from build123d import *

# Parameters (mm, degrees)
SKETCH1_W           = 169
SKETCH1_H           = 4
BOSS_EXTRUDE1_DEPTH = 109
SKETCH3_W           = 165
SKETCH3_H           = 105
CUT_EXTRUDE1_DEPTH  = 1.5
SKETCH4_W           = 151
SKETCH4_H           = 91
CUT_EXTRUDE2_DEPTH  = 5
SKETCH5_W           = 84.5
SKETCH5_H           = 1.5
CUT_EXTRUDE3_DEPTH  = 2


with BuildPart() as part:
    # Sketch1 → Boss-Extrude1 (new body)
    with BuildSketch(Plane.XY):
        with Locations((84.5, 2)):
            Rectangle(SKETCH1_W, SKETCH1_H)
    extrude(amount=-BOSS_EXTRUDE1_DEPTH)

    # Sketch3 → Cut-Extrude1 (cut)
    with BuildSketch(Plane.XZ):
        with Locations((84.5, -54.5)):
            Rectangle(SKETCH3_W, SKETCH3_H)
    extrude(amount=-CUT_EXTRUDE1_DEPTH, mode=Mode.SUBTRACT)

    # Sketch4 → Cut-Extrude2 (cut)
    with BuildSketch(Plane(origin=(0, 4, 0), x_dir=(1, 0, 0), z_dir=(0, 1, 0))):
        with Locations((84.5, 54.5)):
            Rectangle(SKETCH4_W, SKETCH4_H)
    extrude(amount=-CUT_EXTRUDE2_DEPTH, mode=Mode.SUBTRACT)

    # Sketch5 → Cut-Extrude3 (cut)
    with BuildSketch(Plane.XY):
        with Locations((84.5, 0.75)):
            Rectangle(SKETCH5_W, SKETCH5_H)
    extrude(amount=-CUT_EXTRUDE3_DEPTH, mode=Mode.SUBTRACT)


solid = part.part
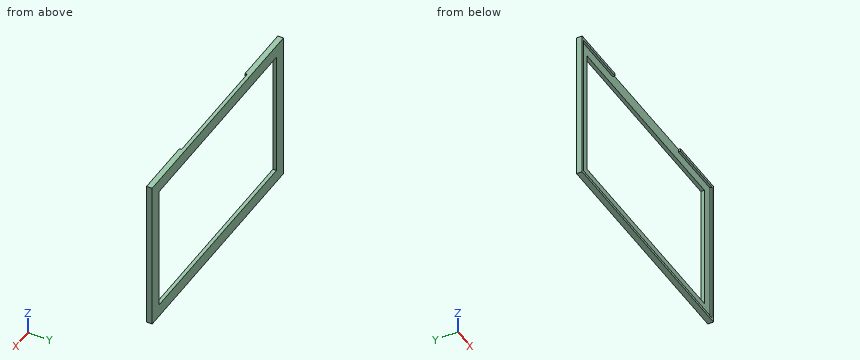
Check sheet for the modelled part. Datum: model origin and axes. Units: mm. Round coordinates to 2 decimals unless told otherwise and drop trailing zeros. Order: outer loops, then holes, each group sorted by start corner. A loop starts at its lowest first (then second) coordinate and runs counter-clockwise, first axis right, second up.
(1) Cross-section at C-C, the plane z = -71. Enter the section's corners in (x, y), and give its area (3 significant figures).
(2) Cross-section at B-B, the plane y = 2.95. Enter the section's corners in (x, z).
(3) Cross-section at D-D, the plane x = 70.5. Enter the section's corners in (y, z).
(4) Cross-section at A-A, the plane x = 146.5. Enter the section's corners in (y, z), and give its area (3 significant figures).
(5) Scan lines: probe 1 along Z at (x, y) = (32, 0.6); probe 2 along Z at (x, y) = (52.5, 2.6); probe 3 along X at (y, z) = (0.35, -90.5). Record each from-to range of solid material in increasing order.
(6) Go/stop test with flat-tipped pins: P1, Ø10, axis at x = 57.5, z = -91, coming from the -Y side; P2, Ø1.2, axis at x = 72, y = 0.5, coming from the +Z side. Record where each tip stops, or that it passes through.
Check sheet entries:
1. outline: (0, 0) - (2, 0) - (2, 1.5) - (9, 1.5) - (9, 4) - (0, 4) - close; (160, 1.5) - (167, 1.5) - (167, 0) - (169, 0) - (169, 4) - (160, 4) - close
1. area: 51.0 mm2
2. outline: (0, -109) - (169, -109) - (169, 0) - (0, 0) - close; hole (9, -100) - (160, -100) - (160, -9) - (9, -9) - close
3. outline: (0, -109) - (4, -109) - (4, -100) - (1.5, -100) - (1.5, -107) - (0, -107) - close; (1.5, -9) - (4, -9) - (4, 0) - (1.5, 0) - close
4. outline: (0, -109) - (4, -109) - (4, -100) - (1.5, -100) - (1.5, -107) - (0, -107) - close; (0, -2) - (1.5, -2) - (1.5, -9) - (4, -9) - (4, 0) - (0, 0) - close
4. area: 51.0 mm2
5. probe 1: z = -109 to -107, -2 to 0
5. probe 2: z = -109 to -100, -9 to 0
5. probe 3: x = 0 to 2, 167 to 169
6. P1: passes through
6. P2: stops at z = -107
